Work out the finished part from the listing and answer in its coordinate system (mm). Face numbers are marked on the shaded views. Coordinates: 2 decimals unless noted, no trailing zeros. One line per question, with ' | ' between items.
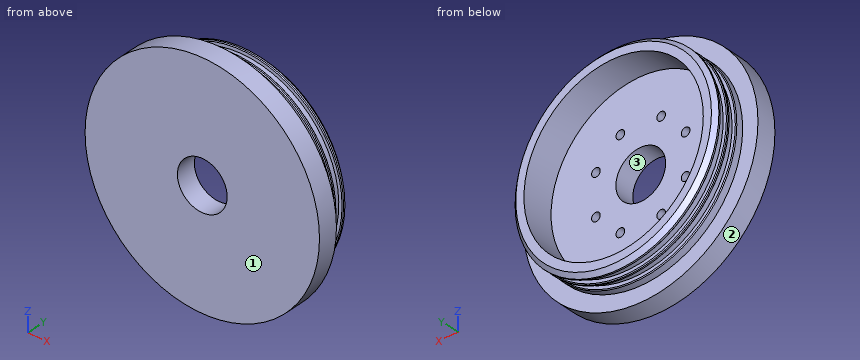
```python
from build123d import *

# Parameters (mm, degrees)
SKETCH1_R                            = 36.5125
EXTRUDE1_DEPTH                       = 3.175
EXTRUDE1_DEPTH_BACK                  = 3.175
SKETCH2_R                            = 31.75
EXTRUDE2_DEPTH                       = 10.16
SKETCH4_W                            = 1.27
SKETCH4_H                            = 2.3622
SKETCH5_R                            = 27.94
CUT_EXTRUDE1_DEPTH                   = 10.16
CHAMFER1_SIZE                        = 1.27
CHAMFER2_SIZE                        = 0.254
TAP_DRILL_FOR_6_TAP1_D               = 2.7051
TAP_DRILL_FOR_6_TAP1_DEPTH           = 3.302
TAP_DRILL_FOR_6_TAP1_TIP             = 0.81269403
TAP_DRILL_FOR_6_TAP1_ON_FACE_2_D     = 2.7051
TAP_DRILL_FOR_6_TAP1_ON_FACE_2_DEPTH = 3.302
TAP_DRILL_FOR_6_TAP1_ON_FACE_2_TIP   = 0.81269403


with BuildPart() as part:
    # Sketch1 → Extrude1 (new body, two sides)
    with BuildSketch(Plane(origin=(0, 0, 0), x_dir=(1, 0, 0), z_dir=(0, 1, 0))) as extrude1_sk:
        Circle(SKETCH1_R)
    extrude(amount=EXTRUDE1_DEPTH)
    extrude(extrude1_sk.sketch, amount=-EXTRUDE1_DEPTH_BACK)

    # Sketch2 → Extrude2 (add)
    with BuildSketch(Plane(origin=(0, 3.175, 0), x_dir=(-1, 0, 0), z_dir=(0, 1, 0))):
        Circle(SKETCH2_R)
    extrude(amount=EXTRUDE2_DEPTH)

    # Sketch4 → Cut-Revolve7 (revolve, cut)
    with BuildSketch(Plane(origin=(0, 0, 0), x_dir=(0, 0, -1), z_dir=(1, 0, 0))):
        with Locations((-31.115, 10.122310801)):
            Rectangle(SKETCH4_W, SKETCH4_H)
        with Locations((-31.115, 6.799968424)):
            Rectangle(SKETCH4_W, SKETCH4_H)
    revolve(axis=Axis((0, -3.175, 0), (0, 1, 0)), mode=Mode.SUBTRACT)

    # Sketch5 → Cut-Extrude1 (cut)
    with BuildSketch(Plane(origin=(0, 13.335, 0), x_dir=(-1, 0, 0), z_dir=(0, 1, 0))):
        Circle(SKETCH5_R)
    extrude(amount=-CUT_EXTRUDE1_DEPTH, mode=Mode.SUBTRACT)

    # Chamfer1
    chamfer1_edges = [part.edges().sort_by_distance(p)[0] for p in [
        (31.75, 13.335, 0),
    ]]
    chamfer(chamfer1_edges, length=CHAMFER1_SIZE)

    # Sketch9 → M14 Clearance Hole1 (revolve, cut)
    with BuildSketch(Plane(origin=(0, -3.175, 0), x_dir=(0, 0, -1), z_dir=(1, 0, 0))):
        Polygon((0, 0), (0, 334.856669797), (7.75, 330.2), (7.75, 0), align=None)
    revolve(axis=Axis((0, -9.525, 0), (0, 1, 0)), mode=Mode.SUBTRACT)

    # Chamfer2
    chamfer2_edges = [part.edges().sort_by_distance(p)[0] for p in [
        (31.75, 11.303410801, 0),
        (31.75, 8.941210801, 0),
        (31.75, 7.981068424, 0),
        (31.75, 5.618868424, 0),
    ]]
    chamfer(chamfer2_edges, length=CHAMFER2_SIZE)

    # Tap Drill for _6 Tap1
    with Locations(Plane(origin=(-6.35, 3.175, 13.97), x_dir=(0, 0, 1), z_dir=(0, 1, 0))):
        with Locations((0, 0), (0, 12.7), (-7.62, 20.32), (-20.32, 20.32), (-27.94, 12.7), (-27.94, 0), (-20.32, -7.62), (-7.62, -7.62), (-13.97, 6.35)):
            Hole(TAP_DRILL_FOR_6_TAP1_D / 2, depth=TAP_DRILL_FOR_6_TAP1_DEPTH)
            with Locations((0, 0, -(TAP_DRILL_FOR_6_TAP1_DEPTH + TAP_DRILL_FOR_6_TAP1_TIP / 2))):  # 118° drill point
                Cone(0, TAP_DRILL_FOR_6_TAP1_D / 2, TAP_DRILL_FOR_6_TAP1_TIP, mode=Mode.SUBTRACT)

    # Tap Drill for _6 Tap1 on face 2
    with Locations(Plane.ZX):
        with Locations((0, 0)):
            Hole(TAP_DRILL_FOR_6_TAP1_ON_FACE_2_D / 2, depth=TAP_DRILL_FOR_6_TAP1_ON_FACE_2_DEPTH)
            with Locations((0, 0, -(TAP_DRILL_FOR_6_TAP1_ON_FACE_2_DEPTH + TAP_DRILL_FOR_6_TAP1_ON_FACE_2_TIP / 2))):  # 118° drill point
                Cone(0, TAP_DRILL_FOR_6_TAP1_ON_FACE_2_D / 2, TAP_DRILL_FOR_6_TAP1_ON_FACE_2_TIP, mode=Mode.SUBTRACT)


solid = part.part
```
1) Find section A-A (y = 1.75). State how many separate pieces and enclosed holes the cut face has, plus the area to 3 significant figures.
Check values:
separate pieces: 1 | enclosed holes: 9 | area: 3,950 mm^2
2) Flat-ended cylindrical pins translate along their axes: pin 1 (2.5 mm diameter, centred on x = -6.35, z = -13.97, fed in from +Y); pin 2 (19 mm diameter, centred on x = -3, z = -15, fed in from +Y) (3 decimals); pin 3 (1.5 mm diameter, centred on y = 0.5, z = 4, fed in from +X); pin 4 (12 mm diameter, centred on x = 24.5, z = -9.5, fed in from +Y) (3 decimals). Find the tip coordinate at first contact, or state that the pin passes through.
Check values:
pin 1: stops at y = -0.19 | pin 2: stops at y = 3.175 | pin 3: stops at x = 36.37 | pin 4: stops at y = 13.335
3) Find the intervals of material crossed by line 1 along X through (y, z) = (1.2, -6.35); line 2 along Y through (x, z) = (8, -23.5) (3 decimals); line 3 along Y through (x, z) = (28, 14) (3 decimals), in increasing order.
Check values:
line 1: x = -35.96 to -15.32, -12.62 to -4.44, 4.44 to 12.62, 15.32 to 35.96 | line 2: y = -3.175 to 3.175 | line 3: y = -3.175 to 5.619, 7.981 to 8.941, 11.303 to 12.51
4) The mould has two halves that part along Z. Classify the marked faces 1, 2 and 3: released by +Z, released by -Z, zero draft, split by the parting line, or undercut.
Check values:
face 1: zero draft | face 2: split by the parting line | face 3: undercut
